from build123d import *

# Parameters (mm, degrees)
CROQUIS1_W              = 14
CROQUIS1_H              = 10
SALIENTE_EXTRUIR1_DEPTH = 1.5
CROQUIS2_R              = 2.65
CROQUIS2_W              = 20.5
CROQUIS2_H              = 12
CORTAR_EXTRUIR1_DEPTH   = 10


with BuildPart() as part:
    # Croquis1 → Saliente-Extruir1 (new, symmetric)
    with BuildSketch(Plane(origin=(0, 0, 0), x_dir=(1, 0, 0), z_dir=(0, 1, 0))):
        with BuildLine():
            ThreePointArc((54.607006458, 65.138888889), (52.033105226, 60.124324936), (49, 55.373420614))
            Line((49, 55.373420614), (49, -27))
            Line((49, -27), (49, -37))
            Line((49, -37), (49, -65))
            Line((49, -65), (35, -65))
            Line((35, -65), (35, -37))
            Line((35, -37), (35, -27))
            Line((35, -27), (35, 41.266028276))
            ThreePointArc((35, 41.266028276), (0, 30), (-35, 41.266028276))
            Line((-35, 41.266028276), (-35, -27))
            Line((-35, -27), (-35, -37))
            Line((-35, -37), (-35, -65))
            Line((-35, -65), (-49, -65))
            Line((-49, -65), (-49, -37))
            Line((-49, -37), (-49, -27))
            Line((-49, -27), (-49, 55.373420614))
            ThreePointArc((-49, 55.373420614), (-52.033105226, 60.124324936), (-54.607006458, 65.138888889))
            ThreePointArc((-54.607006458, 65.138888889), (-35.940259119, -77.027902571), (85, 0))
            ThreePointArc((85, 0), (77.027902571, 35.940259119), (54.607006458, 65.138888889))
        make_face()
        with BuildLine():
            Line((35, 77), (35, 77.459666924))
            ThreePointArc((35, 77.459666924), (0, 85), (-35, 77.459666924))
            Line((-35, 77.459666924), (-35, 77))
            Line((-35, 77), (-35, 41.266028276))
            ThreePointArc((-35, 41.266028276), (0, 30), (35, 41.266028276))
            Line((35, 41.266028276), (35, 77))
        make_face()
        with BuildLine():
            Line((-49, 55.373420614), (-49, 69.455021417))
            ThreePointArc((-49, 69.455021417), (-51.848434854, 67.35532498), (-54.607006458, 65.138888889))
            ThreePointArc((-54.607006458, 65.138888889), (-52.033105226, 60.124324936), (-49, 55.373420614))
        make_face()
        with BuildLine():
            Line((35, 115), (49, 115))
            Line((49, 115), (49, 87))
            Line((49, 87), (49, 77))
            Line((49, 77), (49, 69.455021417))
            ThreePointArc((49, 69.455021417), (51.848434854, 67.35532498), (54.607006458, 65.138888889))
            ThreePointArc((54.607006458, 65.138888889), (58.636253238, 77.280337809), (60, 90))
            ThreePointArc((60, 90), (-12.719662191, 148.636253238), (-54.607006458, 65.138888889))
            ThreePointArc((-54.607006458, 65.138888889), (-51.848434854, 67.35532498), (-49, 69.455021417))
            Line((-49, 69.455021417), (-49, 77))
            Line((-49, 77), (-49, 87))
            Line((-49, 87), (-49, 115))
            Line((-49, 115), (-35, 115))
            Line((-35, 115), (-35, 87))
            Line((-35, 87), (-35, 77.459666924))
            ThreePointArc((-35, 77.459666924), (0, 85), (35, 77.459666924))
            Line((35, 77.459666924), (35, 87))
            Line((35, 87), (35, 115))
        make_face()
        with BuildLine():
            ThreePointArc((54.607006458, 65.138888889), (51.848434854, 67.35532498), (49, 69.455021417))
            Line((49, 69.455021417), (49, 55.373420614))
            ThreePointArc((49, 55.373420614), (52.033105226, 60.124324936), (54.607006458, 65.138888889))
        make_face()
        with Locations((-42, -32)):
            Rectangle(CROQUIS1_W, CROQUIS1_H)
        with Locations((42, -32)):
            Rectangle(CROQUIS1_W, CROQUIS1_H)
        with Locations((42, 82)):
            Rectangle(CROQUIS1_W, CROQUIS1_H)
        with Locations((-42, 82)):
            Rectangle(CROQUIS1_W, CROQUIS1_H)
    extrude(amount=SALIENTE_EXTRUIR1_DEPTH, both=True)

    # Croquis2 → Cortar-Extruir1 (cut)
    with BuildSketch(Plane.XZ.offset(1.5)):
        with Locations(Location((-20, -120, 0), (0, 0, 270))):
            Circle(CROQUIS2_R)
        with Locations(Location((20, -120, 0), (0, 0, 270))):
            Circle(CROQUIS2_R)
        with Locations((0, 51)):
            Rectangle(CROQUIS2_W, CROQUIS2_H)
    extrude(amount=-CORTAR_EXTRUIR1_DEPTH, mode=Mode.SUBTRACT)


solid = part.part
Build history of the part. All positions in model axes, mm. Coordinates: 2 decimals unless noted, no trailing zeros. Order: outer loops, then holes, each group sorted by start corner. A loop starts at its lowest first (then second) coordinate and runs counter-clockwise, first axis right, second up. Notation, with made-up numbers: (85, 33) - (93, 33) arc R14 ccw to (93, 39) - close; hole circle Ø2 at (61, 11.5). An arc over 180 degrees is marked (long way). Write each question's results on one line, items separated by ' | '. Start each with the question number.
Item 1: Band-saw the part on A-A on z = 0. Write the cut outline in (x, y), and give its area (3 significant figures).
Item 2: Mould opens along Z. For faces 1 (the face through (-1, -1.5, -34)), 2 (the face through (20.796, -0.021, -122.528)) say: released by +Z, released by -Z, zero draft, split by the parting line, or undercut.
Item 3: Wall check: probe 1 along X at (y, z) = (0.35, 2); probe 2 along Z at (x, y) = (44, 0.75); probe 3 along X at (y, z) = (0.5, -39.5). Give the ranges that are in metal, low to high. Write a range as [from, to].
Item 4: Flat gauge pins, fed straight in: pin 1 (0.9 mm diameter, centred on x = -44.5, y = 0.5, fed in from +Z); pin 2 (0.9 mm diameter, centred on x = -45, y = 0, fed in from -Z); pin 3 (1.5 mm diameter, centred on y = -0.5, z = 37.5, fed in from -X); pin 4 (5 mm diameter, centred on x = -20, z = -120, fed in from +Y). Where does each tip first touch, or does it go through?
Item 5: Band-saw the part on B-B on x = 0. Write the cut outline in (y, z), and give its area (3 significant figures).
Item 6: Band-saw the part on D-D on z = -90. Write the cut outline in (x, y), and give its area (3 significant figures).
Item 7: Band-saw the part on C-C on y = -0.95. State how many separate pieces and enclosed holes the cut face has, and give its area (3 significant figures).
Numbers:
1) outline: (-85, -1.5) - (-49, -1.5) - (-49, 1.5) - (-85, 1.5) - close; (-35, -1.5) - (35, -1.5) - (35, 1.5) - (-35, 1.5) - close; (49, -1.5) - (85, -1.5) - (85, 1.5) - (49, 1.5) - close | area: 426 mm^2
2) face 1: zero draft | face 2: undercut
3) probe 1: [-84.98, -49], [-35, 35], [49, 84.98] | probe 2: [-130.79, -115], [-87, -77], [27, 37], [65, 72.73] | probe 3: [-75.26, -49], [-35, 35], [49, 75.26]
4) pin 1: z = 72.7 | pin 2: z = -130.19 | pin 3: x = -76.64 | pin 4: through
5) outline: (-1.5, -150) - (1.5, -150) - (1.5, 45) - (-1.5, 45) - close; (-1.5, 57) - (1.5, 57) - (1.5, 85) - (-1.5, 85) - close | area: 669 mm^2
6) outline: (-60, -1.5) - (-49, -1.5) - (-49, 1.5) - (-60, 1.5) - close; (-35, -1.5) - (35, -1.5) - (35, 1.5) - (-35, 1.5) - close; (49, -1.5) - (60, -1.5) - (60, 1.5) - (49, 1.5) - close | area: 276 mm^2
7) separate pieces: 1 | enclosed holes: 9 | area: 25,000 mm^2
